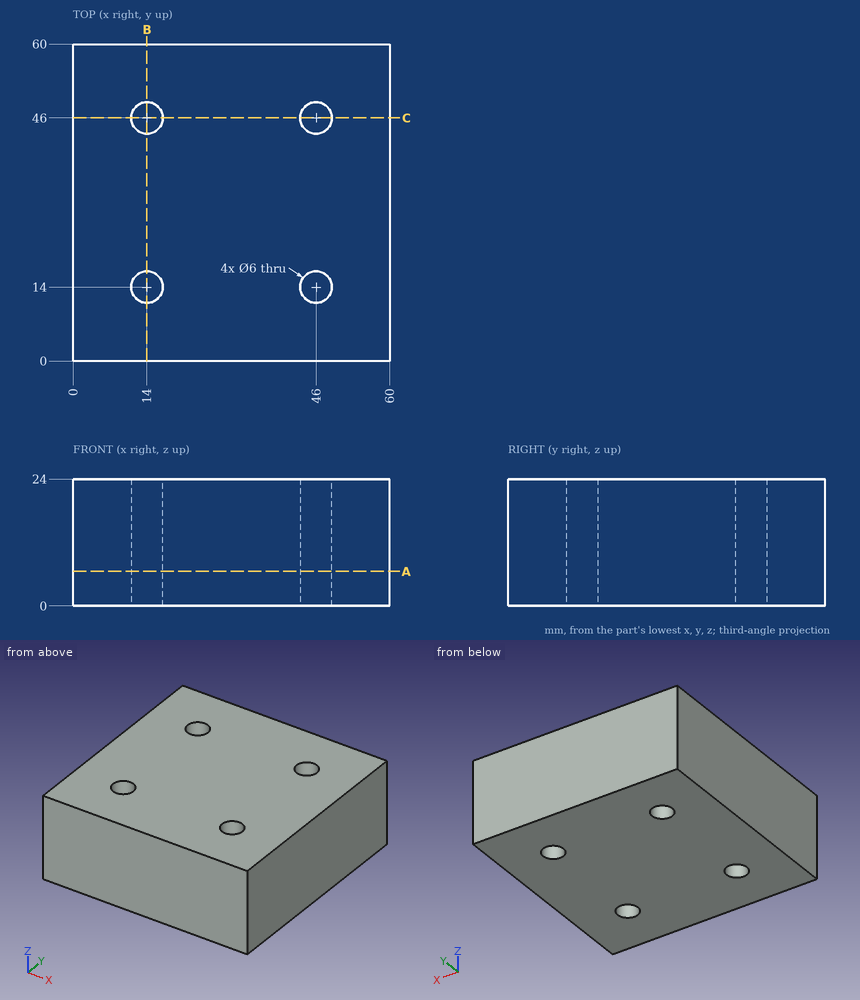
Can you work these out from the drawing? Everything is in mm from the part's minimum corner. Round coordinates to 2 decimals unless told otherwise and drop trailing zeros. Loops run counter-clockwise (first coordinate to the right, second up) from the corner with the lowest first, then second, coordinate; pieces in that order, holes last. Notation, with made-up numbers: (55.5, 3.25) -> (74.5, 3.25) arc R21 cw to (74.5, 41.25) -> close; hole circle Ø11 at (50.5, 78.5). An arc over 180 degrees is marked (long way). One line per question, with ' | ' between items.
(1) If I drill on probe 1 along X at (y, z) = (14, 14.25); probe 2 along X at (y, z) = (12.5, 3), over which ranges is the centre line in solid material (lowest first)?
Model answer:
probe 1: x = 0 to 11, 17 to 43, 49 to 60 | probe 2: x = 0 to 11.4, 16.6 to 43.4, 48.6 to 60
(2) For pin 1 Ø5 at (x, y) = (46, 46) entering from +Z, with a flat end and sliding along its axis, tell me the tip position at first contact or that it passes through.
Model answer:
pin 1: passes through
(3) If we section it at A-A on z = 6.5: List the corners of the cut face in (x, y) for me, and give its area (3 significant figures).
Model answer:
outline: (0, 0) -> (60, 0) -> (60, 60) -> (0, 60) -> close; hole circle Ø6 at (14, 14); hole circle Ø6 at (14, 46); hole circle Ø6 at (46, 14); hole circle Ø6 at (46, 46) | area: 3,490 mm^2
(4) If we section it at B-B on x = 14: List the corners of the cut face in (y, z) for me.
Model answer:
outline: (0, 0) -> (11, 0) -> (11, 24) -> (0, 24) -> close; (17, 0) -> (43, 0) -> (43, 24) -> (17, 24) -> close; (49, 0) -> (60, 0) -> (60, 24) -> (49, 24) -> close
